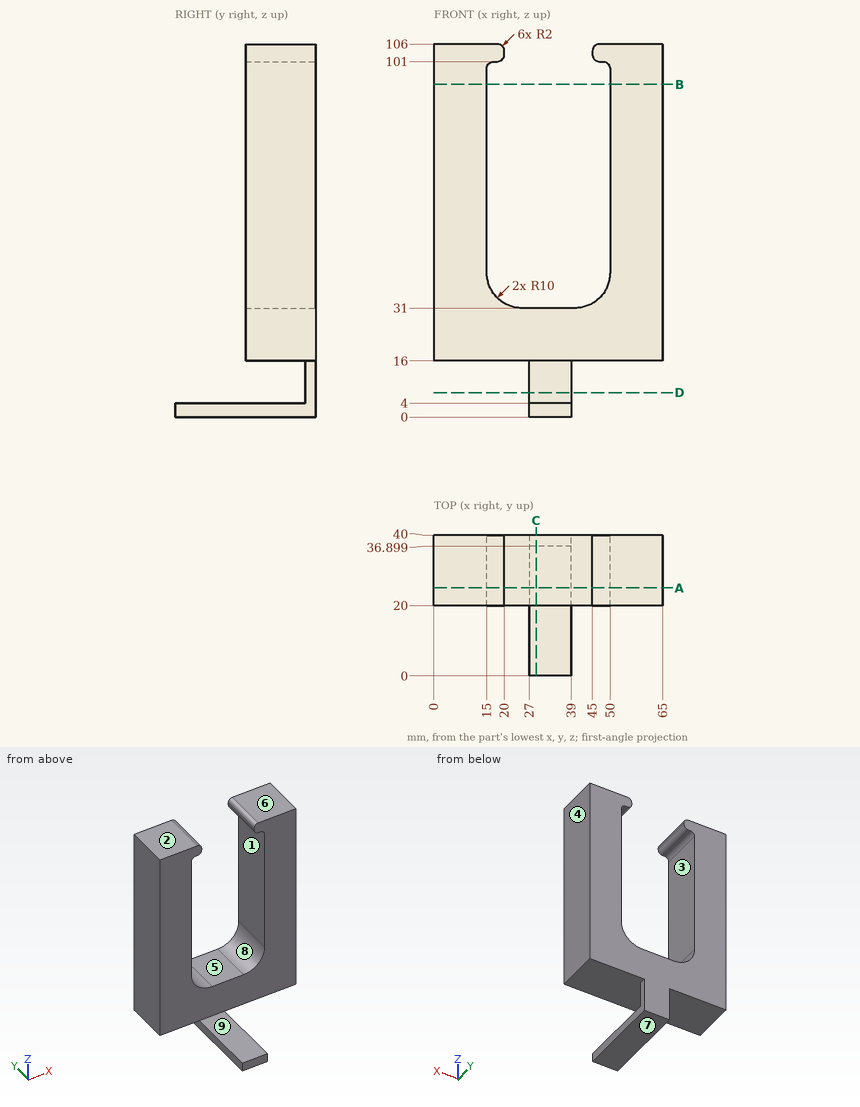
Geometry: see drawing. Coordinates: mm, zero at the bounding-box minimum. A direction names the side the tool comes from. Give positions to 0.01 mm unless a question says otherwise; leave off trailing zeros. Loops run counter-clockwise (first coordinate to the right, second up) from the corner with the lowest first, then second, coordinate; pieces in that order, holes last. Notation, with made-up numbers: (17.5, 83) -> (54.5, 83) arc R27 ccw to (54.5, 104) -> close; hole circle Ø9 at (71, 18). An arc over 180 degrees is marked (long way). Answer as a JSON object with one key per item and string values. Group by question number.
Item 1: Pin query (flat end, axial travel): P1, Ø7.5, axis at x = 36, y = 25.5, coming from the +Z side; P2, Ø9.5, axis at x = 34.5, y = 10.5, coming from the +Z side; P3, Ø10, axis at x = 14, y = 31, coming from the -Z side. Return the tip coordinate at first contact, or that it passes through.
Item 2: Cut plane C-C, the plane x = 29. Return the cut outline in (y, z), and give its area (3 significant figures).
Item 3: Cut plane D-D, the plane z = 7. Return the cut outline in (x, y).
Item 4: Pull-direction query (Z, two-part tool) for the marked faces 1, 2, 3 and 4; classes: released by +Z, released by -Z, zero draft, split by the parting line, or undercut.
Item 5: Line query: probe 1 along X at (y, z) = (25, 97); probe 2 along Z at (x, y) = (34, 28.5); probe 3 along Z at (x, y) = (16, 20.5). Output: solid intervals per line, ascending.
Item 6: Cut plane B-B, the plane z = 94.5. Return the cut outline in (x, y).
Item 7: Reachability of the marked faces 5, 6, 7, 8 and 9 from +Z, -Z, +X, -X, +Y, -Y: full face, straight path, thin tool, end or side. Return the list, or none.
Item 8: Cut plane A-A, the plane y = 25. Return the cut outline in (x, z).
Checks:
{
 "1": {"P1": "stops at z = 31", "P2": "stops at z = 4", "P3": "stops at z = 16"},
 "2": {"outline": "(0, 0) -> (40, 0) -> (40, 31) -> (20, 31) -> (20, 16) -> (36.9, 16) -> (36.9, 4) -> (0, 4) -> close", "area": "497 mm²"},
 "3": {"outline": "(27, 36.9) -> (39, 36.9) -> (39, 40) -> (27, 40) -> close"},
 "4": {"face 1": "undercut", "face 2": "released by +Z", "face 3": "undercut", "face 4": "zero draft"},
 "5": {"probe 1": "x = 0 to 15, 50 to 65", "probe 2": "z = 0 to 4, 16 to 31", "probe 3": "z = 16 to 36.64, 100.73 to 106"},
 "6": {"outline": "(0, 20) -> (15, 20) -> (15, 40) -> (0, 40) -> close; (50, 20) -> (65, 20) -> (65, 40) -> (50, 40) -> close"},
 "7": {"face 5": "+Z, +Y, -Y", "face 6": "+Z, +X, -X, +Y, -Y", "face 7": "-Z, +X, -X, +Y, -Y", "face 8": "+Y, -Y", "face 9": "+X, -X, -Y"},
 "8": {"outline": "(0, 16) -> (65, 16) -> (65, 106) -> (47, 106) arc R2 ccw to (45, 104) -> (45, 103) arc R2 ccw to (47, 101) -> (48, 101) arc R2 cw to (50, 99) -> (50, 41) arc R10 cw to (40, 31) -> (25, 31) arc R10 cw to (15, 41) -> (15, 99) arc R2 cw to (17, 101) -> (18, 101) arc R2 ccw to (20, 103) -> (20, 104) arc R2 ccw to (18, 106) -> (0, 106) -> close; (27, 0) -> (39, 0) -> (39, 4) -> (27, 4) -> close"}
}
